Input: part model. Units: mm. Frame: model coordinates. Round coordinates to 2 decimals unless told otherwise and drop trailing zeros. Write each loop counter-clockwise with the first axis right and the second up, starting at its lowest first coordinate (ties: lowest second). Pieces come first, ordered by that corner, then holes. Notation, with made-up numbers: (63, 84.5) -> (81, 84.5) arc R20 cw to (81, 104.5) -> close; hole circle Ø6 at (-6.75, 67.5). An arc over 180 degrees is marked (long way). Use CSV: the item, a comma, the result in double quotes.
```python
from build123d import *

# Parameters (mm, degrees)
CYLINDER115_R       = 1.8
CYLINDER115_DEPTH   = 10
ARRAY001018_Y_COUNT = 3
ARRAY001018_Y_PITCH = 10
CYLINDER034_R       = 0.8
CYLINDER034_DEPTH   = 30
ARRAY001017_Y_COUNT = 2
ARRAY001017_Y_PITCH = 9
BOX013_W            = 11
BOX013_H            = 50
BOX013_DEPTH        = 3
FILLET006_R         = 3


with BuildPart() as bolt_hole_array:
    # Cylinder115 → Cylinder115 (new body)
    with BuildSketch(Plane.XY):
        Circle(CYLINDER115_R)
    extrude(amount=CYLINDER115_DEPTH)

    # Array001018 Y: bolt hole array ×3


with BuildPart() as bolt_hole_array_1:
    add(bolt_hole_array.part)
    with Locations(*[(0, i * ARRAY001018_Y_PITCH, 0) for i in range(1, ARRAY001018_Y_COUNT)]):
        add(bolt_hole_array.part)


with BuildPart() as bolt_hole_array_2:
    # Array001018 placement: moved
    add(bolt_hole_array_1.part.moved(Location((5.5, 25, 0))))


with BuildPart() as endstop_hole_fusion:
    # Cylinder034 → Cylinder034 (new body)
    with BuildSketch(Plane.XY):
        Circle(CYLINDER034_R)
    extrude(amount=CYLINDER034_DEPTH)

    # Array001017 Y: endstop hole fusion ×2


with BuildPart() as endstop_hole_fusion_1:
    add(endstop_hole_fusion.part)
    with Locations(*[(0, i * ARRAY001017_Y_PITCH, 0) for i in range(1, ARRAY001017_Y_COUNT)]):
        add(endstop_hole_fusion.part)


with BuildPart() as endstop_hole_fusion_2:
    # Array001017 placement: moved
    add(endstop_hole_fusion_1.part.moved(Location((8, 6, 0))))

    # Fusion015: union bolt hole array
    add(bolt_hole_array_2.part)


with BuildPart() as endstop_base_cut:
    # Box013 → Box013 (new body)
    with BuildSketch(Plane.XY):
        with Locations((5.5, 25)):
            Rectangle(BOX013_W, BOX013_H)
    extrude(amount=BOX013_DEPTH)

    # Fillet006
    fillet006_edges = [endstop_base_cut.edges().sort_by_distance(p)[0] for p in [
        (0, 0, 1.5),
        (0, 50, 1.5),
        (11, 0, 1.5),
        (11, 50, 1.5),
    ]]
    fillet(fillet006_edges, radius=FILLET006_R)

    # Cut010: cut endstop hole fusion
    add(endstop_hole_fusion_2.part, mode=Mode.SUBTRACT)


solid = endstop_base_cut.part
```
Item 1: Section query A-A on y = 15. Return the cut outline in (x, z), plus the area to 3 significant figures.
Worked answers:
outline,"(0, 0) -> (7.2, 0) -> (7.2, 3) -> (0, 3) -> close; (8.8, 0) -> (11, 0) -> (11, 3) -> (8.8, 3) -> close"
area,"28.2 mm²"
Item 2: Pull-direction query (X, two-part tool) for faces 1 (the face through (3, 25, 0)), 2 (the face through (7.2, 15, 1.5)), 3 (the face through (10.1, 0.86, 1.52)); classes: +X half, -X half, draft (parallel to the pull), parting line (faces both ways), or undercut.
Worked answers:
face 1,"draft"
face 2,"undercut"
face 3,"+X half"
Item 3: Section query D-D on y = 45. Return the cut outline in (x, z), plus the area to 3 significant figures.
Worked answers:
outline,"(0, 0) -> (3.7, 0) -> (3.7, 3) -> (0, 3) -> close; (7.3, 0) -> (11, 0) -> (11, 3) -> (7.3, 3) -> close"
area,"22.2 mm²"
Item 4: Line query: line 1 (Y direction, x = 5.5, z = 2.2); line 2 (Y direction, x = 8, z = 2.35); line 3 (X direction, y = 15, z = 2.2). Output: solid intervals per line, ascending.
Worked answers:
line 1,"y = 0 to 23.2, 26.8 to 33.2, 36.8 to 43.2, 46.8 to 50"
line 2,"y = 0 to 5.2, 6.8 to 14.2, 15.8 to 50"
line 3,"x = 0 to 7.2, 8.8 to 11"
Item 5: Section query B-B on x = 5.5. Return the cut outline in (y, z), plus the area to 3 significant figures.
Worked answers:
outline,"(0, 0) -> (23.2, 0) -> (23.2, 3) -> (0, 3) -> close; (26.8, 0) -> (33.2, 0) -> (33.2, 3) -> (26.8, 3) -> close; (36.8, 0) -> (43.2, 0) -> (43.2, 3) -> (36.8, 3) -> close; (46.8, 0) -> (50, 0) -> (50, 3) -> (46.8, 3) -> close"
area,"118 mm²"
Item 6: Section query C-C on z = 1.2. Return the cut outline in (x, y), plus the area to 3 significant figures.
Worked answers:
outline,"(0, 3) arc R3 ccw to (3, 0) -> (8, 0) arc R3 ccw to (11, 3) -> (11, 47) arc R3 ccw to (8, 50) -> (3, 50) arc R3 ccw to (0, 47) -> close; hole circle Ø3.6 at (5.5, 25); hole circle Ø3.6 at (5.5, 35); hole circle Ø3.6 at (5.5, 45); hole circle Ø1.6 at (8, 6); hole circle Ø1.6 at (8, 15)"
area,"508 mm²"
Item 7: First-contact query: pin 1 Ø4 at (x, y) = (5.5, 25) entering from +Z. Flat tip, straight axial feed; report the tip coordinate or a pass-through.
Worked answers:
pin 1,"stops at z = 3"
